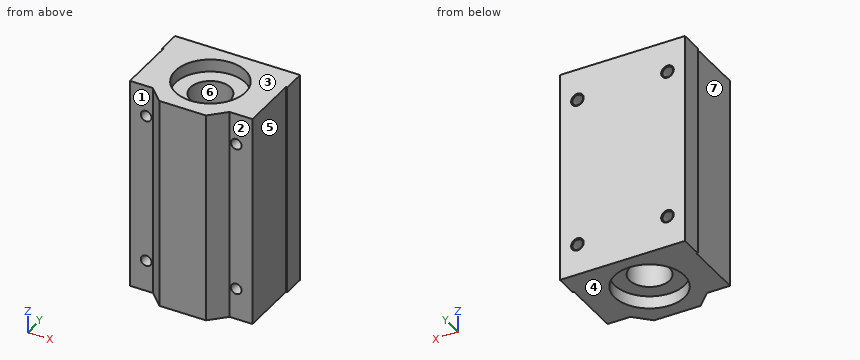
from build123d import *

# Parameters (mm, degrees)
SKETCH_1_R                  = 8
EXTRUDE_1_DEPTH             = 85
SKETCH_2_R                  = 1
CUT_EXTRUDE_1_DEPTH         = 97.603571363
HOLE_WIZARD_M51_D           = 4.2
HOLE_WIZARD_M51_DEPTH       = 14
HOLE_WIZARD_M51_CSINK_D     = 5.05
HOLE_WIZARD_M51_CSINK_ANGLE = 120
HOLE_WIZARD_M51_TIP         = 1.2618073
SKETCH_6_R                  = 2.15
CUT_EXTRUDE_3_DEPTH         = 24
SKETCH_7_R                  = 14
CUT_EXTRUDE_4_DEPTH         = 5
CUT_EXTRUDE_START           = -5
SKETCH_8_R                  = 14
CUT_EXTRUDE_5_DEPTH         = 5


with BuildPart() as part:
    # Эскиз1 → Бобышка-Вытянуть1 (new body)
    with BuildSketch(Plane.XY):
        Polygon((-25, 19), (25, 19), (25, 10), (24.5, 10), (24.5, -13.5), (15.329639, -13.5), (9.329639, -19.5), (-9.329639, -19.5), (-15.329639, -13.5), (-24.5, -13.5), (-24.5, 10), (-25, 10), align=None)
        Circle(SKETCH_1_R, mode=Mode.SUBTRACT)
    extrude(amount=EXTRUDE_1_DEPTH)

    # Эскиз2 → Вырез-Вытянуть1 (cut, through all)
    with BuildSketch(Plane(origin=(0, 19, 0), x_dir=(1, 0, 0), z_dir=(0, 1, 0))):
        with Locations(Location((-18, -12.5, 0), (0, 0, 270))):
            Circle(SKETCH_2_R)
        with Locations(Location((-18, -72.5, 0), (0, 0, 270))):
            Circle(SKETCH_2_R)
        with Locations(Location((18, -72.5, 0), (0, 0, 270))):
            Circle(SKETCH_2_R)
        with Locations(Location((18, -12.5, 0), (0, 0, 270))):
            Circle(SKETCH_2_R)
    extrude(amount=-CUT_EXTRUDE_1_DEPTH, mode=Mode.SUBTRACT)

    # Отверстие обработанное метчиком M51
    with Locations(Plane(origin=(0, 19, 0), x_dir=(-1, 0, 0), z_dir=(0, 1, 0))):
        with Locations((-18, 12.5), (-18, 72.5), (18, 72.5), (18, 12.5)):
            CounterSinkHole(HOLE_WIZARD_M51_D / 2, HOLE_WIZARD_M51_CSINK_D / 2, depth=HOLE_WIZARD_M51_DEPTH, counter_sink_angle=HOLE_WIZARD_M51_CSINK_ANGLE)
            with Locations((0, 0, -(HOLE_WIZARD_M51_DEPTH + HOLE_WIZARD_M51_TIP / 2))):  # 118° drill point
                Cone(0, HOLE_WIZARD_M51_D / 2, HOLE_WIZARD_M51_TIP, mode=Mode.SUBTRACT)

    # Эскиз6 → Вырез-Вытянуть3 (cut)
    with BuildSketch(Plane.XZ.offset(13.5)):
        with Locations(Location((-18, 72.5, 0), (0, 0, 270))):
            Circle(SKETCH_6_R)
        with Locations(Location((18, 72.5, 0), (0, 0, 270))):
            Circle(SKETCH_6_R)
        with Locations(Location((18, 12.5, 0), (0, 0, 270))):
            Circle(SKETCH_6_R)
        with Locations(Location((-18, 12.5, 0), (0, 0, 270))):
            Circle(SKETCH_6_R)
    extrude(amount=-CUT_EXTRUDE_3_DEPTH, mode=Mode.SUBTRACT)

    # Эскиз7 → Вырез-Вытянуть4 (cut)
    with BuildSketch(Plane(origin=(0, 0, 0), x_dir=(-1, 0, 0), z_dir=(0, 0, -1))):
        Circle(SKETCH_7_R)
    extrude(amount=-CUT_EXTRUDE_4_DEPTH, mode=Mode.SUBTRACT)

    # Эскиз8 → Вырез-Вытянуть5 (cut)
    with BuildSketch(Plane.XY.offset(85).offset(CUT_EXTRUDE_START)):
        with Locations(Location((0, 0, 0), (0, 0, 180))):
            Circle(SKETCH_8_R)
    extrude(amount=CUT_EXTRUDE_5_DEPTH, mode=Mode.SUBTRACT)


solid = part.part
The listing builds one solid part. Answer for the finished solid, in the listing's coordinates (mm). Face numbers are marked on the shaded views. A direction names the side the tool comes from. Give positions to 0.01 mm unless a question says otherwise; leave off trailing zeros. Write each loop counter-clockwise with the first axis right and the second up, starting at its lowest first coordinate (ties: lowest second). Pieces come first, ordered by that corner, then holes.
1) For a pull along X with two mould halves and no side action, classify the marked faces 4, 5, 6 and 7 as pulls with the +X half, pulls with the -X half, needs draft (parallel to the pull), parting line crosses it, or undercut.
2) A tool of negligible diameter and unlimited length cuts with its end or side. For the marked faces 1, 2 and 3, from which of +Z, -Z, +X, -X, +Y, -Y can it reach the whole face along a straight path? Write none if from no direction.
3) Section D-D (y = -7) is taken. Write down the section's boundary in (x, z), and give its area (3 significant figures).
4) Section A-A (x = -18) is taken. Write down the section's boundary in (y, z) (3 decimals).
5) Section B-B (z = 72.5) is taken. Count the separate pieces of the cut face and the enclosed holes in it, and give its area (3 significant figures).
6) Find the intervals of material crossed by L1, parallel to X at y = 14, z = 12.5; L2, parallel to Z at x = -17, y = 1; L3, parallel to X at y = 0.5, z = 57.5, in increasing order.
7) Section C-C (z = 8.5) is taken. Write down the section's boundary in (x, y).
8) Given P1, Ø1.5, axis at y = 7.5, z = 73, coming from the +X side; P2, Ø4.5, axis at x = -18.5, z = 72, coming from the -Y side; P3, Ø22.5, axis at x = 0, y = 0, coming from the -Z side, each flat-ended and moving along its own axis, determine where each tip first touches the part or whether it passes through.
Response:
1. face 4: needs draft
1. face 5: pulls with the +X half
1. face 6: undercut
1. face 7: pulls with the -X half
2. face 1: +Z, -Z, -X, -Y
2. face 2: +Z, -Z, +X, -Y
2. face 3: +Z, +X, -X, +Y, -Y
3. outline: (-24.5, 0) - (-12.12, 0) - (-12.12, 5) - (-3.87, 5) - (-3.87, 80) - (-12.12, 80) - (-12.12, 85) - (-24.5, 85) - close; (3.87, 5) - (12.12, 5) - (12.12, 0) - (24.5, 0) - (24.5, 85) - (12.12, 85) - (12.12, 80) - (3.87, 80) - close; hole circle Ø4.3 at (-18, 12.5); hole circle Ø4.3 at (-18, 72.5); hole circle Ø4.3 at (18, 12.5); hole circle Ø4.3 at (18, 72.5)
3. area: 3,280 mm2
4. outline: (-13.5, 0) - (19, 0) - (19, 9.975) - (18.755, 10.4) - (10.5, 10.4) - (10.5, 10.35) - (-13.5, 10.35) - close; (-13.5, 14.65) - (10.5, 14.65) - (10.5, 14.6) - (18.755, 14.6) - (19, 15.025) - (19, 69.975) - (18.755, 70.4) - (10.5, 70.4) - (10.5, 70.35) - (-13.5, 70.35) - close; (-13.5, 74.65) - (10.5, 74.65) - (10.5, 74.6) - (18.755, 74.6) - (19, 75.025) - (19, 85) - (-13.5, 85) - close
5. separate pieces: 3
5. enclosed holes: 1
5. area: 1,270 mm2
6. L1: x = -25 to -20.1, -15.9 to 15.9, 20.1 to 25
6. L2: z = 0 to 10.6, 14.4 to 70.6, 74.4 to 85
6. L3: x = -24.5 to -7.98, 7.98 to 24.5
7. outline: (-25, 10) - (-24.5, 10) - (-24.5, -13.5) - (-15.33, -13.5) - (-9.33, -19.5) - (9.33, -19.5) - (15.33, -13.5) - (24.5, -13.5) - (24.5, 10) - (25, 10) - (25, 19) - (-25, 19) - close; hole circle Ø16 at (0, 0)
8. P1: stops at x = 24.5
8. P2: stops at y = -13.5
8. P3: stops at z = 5
